Part model, mm, in its own coordinate system. A direction names the side the tool comes from. Round coordinates to 2 decimals unless told otherwise and drop trailing zeros. Loops run counter-clockwise (first coordinate to the right, second up) from the corner with the lowest first, then second, coordinate; pieces in that order, holes last.
from build123d import *

# Parameters (mm, degrees)
SKETCH_1_W           = 30
SKETCH_1_H           = 14.828427124
EXTRUDE_2_DEPTH      = 10
CUT_EXTRUDE_9_DEPTH  = 15
CUT_EXTRUDE_10_DEPTH = 30
CUT_EXTRUDE_11_DEPTH = 31
CUT_EXTRUDE_12_DEPTH = 40
SKETCH_1_15_R        = 6
CUT_EXTRUDE_13_DEPTH = 17
CUT_EXTRUDE_17_DEPTH = 97
CUT_EXTRUDE_18_DEPTH = 285
CUT_EXTRUDE_20_DEPTH = 202
CUT_EXTRUDE_21_DEPTH = 202
CUT_EXTRUDE_22_DEPTH = 95


with BuildPart() as part:
    # Sketch 1 → Extrude 2 (new body)
    with BuildSketch(Plane.XY):
        with Locations((7.585786438, 0)):
            Rectangle(SKETCH_1_W, SKETCH_1_H)
    extrude(amount=EXTRUDE_2_DEPTH)

    # Sketch 1_11 → Cut-Extrude 9 (cut)
    with BuildSketch(Plane.XY):
        with BuildLine():
            Line((0, -2), (0, 0))
            Line((0, 0), (-6, 0))
            ThreePointArc((-6, 0), (-4.242640687, -4.242640687), (0, -6))
            ThreePointArc((0, -6), (3.464101615, -4.898979486), (5.656854249, -2))
            Line((5.656854249, -2), (0, -2))
        make_face()
    extrude(amount=CUT_EXTRUDE_9_DEPTH, mode=Mode.SUBTRACT)

    # Sketch 1_12 → Cut-Extrude 10 (cut)
    with BuildSketch(Plane.XY):
        with BuildLine():
            Line((-6, 0), (0, 0))
            Line((0, 0), (0, 2))
            Line((0, 2), (0, 6))
            ThreePointArc((0, 6), (-4.242640687, 4.242640687), (-6, 0))
        make_face()
    extrude(amount=CUT_EXTRUDE_10_DEPTH, mode=Mode.SUBTRACT)

    # Sketch 1_13 → Cut-Extrude 11 (cut)
    with BuildSketch(Plane.XY):
        with BuildLine():
            Line((0, 2), (0, 0))
            Line((0, 0), (6, 0))
            ThreePointArc((6, 0), (5.913591358, 1.014611872), (5.656854249, 2))
            Line((5.656854249, 2), (0, 2))
        make_face()
    extrude(amount=CUT_EXTRUDE_11_DEPTH, mode=Mode.SUBTRACT)

    # Sketch 1_14 → Cut-Extrude 12 (cut)
    with BuildSketch(Plane.XY):
        with BuildLine():
            Line((6, 0), (0, 0))
            Line((0, 0), (0, -2))
            Line((0, -2), (5.656854249, -2))
            ThreePointArc((5.656854249, -2), (5.913591358, -1.014611872), (6, 0))
        make_face()
    extrude(amount=CUT_EXTRUDE_12_DEPTH, mode=Mode.SUBTRACT)

    # Sketch 1_15 → Cut-Extrude 13 (cut)
    with BuildSketch(Plane.XY):
        with Locations(Location((0, 0, 0), (0, 0, 180))):
            Circle(SKETCH_1_15_R)
    extrude(amount=CUT_EXTRUDE_13_DEPTH, mode=Mode.SUBTRACT)

    # Sketch 1_19 → Cut-Extrude 17 (cut)
    with BuildSketch(Plane.XY):
        with BuildLine():
            ThreePointArc((5.656854249, 2), (5.913591358, 1.014611872), (6, 0))
            Line((6, 0), (6, 2))
            Line((6, 2), (5.656854249, 2))
        make_face()
        Polygon((6, 2), (6, 0), (7, 0), (7, 1), (7, 2), align=None)
        Polygon((7, 0), (6, 0), (6, -2), (7, -2), (7, -1), align=None)
        with BuildLine():
            Line((6, -2), (6, 0))
            ThreePointArc((6, 0), (5.913591358, -1.014611872), (5.656854249, -2))
            Line((5.656854249, -2), (6, -2))
        make_face()
    extrude(amount=CUT_EXTRUDE_17_DEPTH, mode=Mode.SUBTRACT)

    # Sketch 1_20 → Cut-Extrude 18 (cut)
    with BuildSketch(Plane.XY):
        with BuildLine():
            ThreePointArc((7.414213562, 7.414213562), (9.005239827, 5.370919954), (10.046946078, 3))
            Line((10.046946078, 3), (18, 3))
            Line((18, 3), (18, 2))
            Line((18, 2), (18, 1))
            Line((18, 1), (18, -1))
            Line((18, -1), (18, -2))
            Line((18, -2), (18, -3))
            Line((18, -3), (10.046946078, -3))
            ThreePointArc((10.046946078, -3), (9.005239827, -5.370919954), (7.414213562, -7.414213562))
            Line((7.414213562, -7.414213562), (22.585786438, -7.414213562))
            Line((22.585786438, -7.414213562), (22.585786438, 7.414213562))
            Line((22.585786438, 7.414213562), (7.414213562, 7.414213562))
        make_face()
    extrude(amount=CUT_EXTRUDE_18_DEPTH, mode=Mode.SUBTRACT)

    # Sketch 1_22 → Cut-Extrude 20 (cut)
    with BuildSketch(Plane.XY):
        with BuildLine():
            ThreePointArc((10.485281374, 0), (10.473325852, -0.500570761), (10.437486551, -1))
            Line((10.437486551, -1), (18, -1))
            Line((18, -1), (18, 1))
            Line((18, 1), (10.437486551, 1))
            ThreePointArc((10.437486551, 1), (10.473325852, 0.500570761), (10.485281374, 0))
        make_face()
    extrude(amount=CUT_EXTRUDE_20_DEPTH, mode=Mode.SUBTRACT)

    # Sketch 2 → Cut-Extrude 21 (cut)
    with BuildSketch(Plane.XZ.offset(3)):
        with BuildLine():
            ThreePointArc((14.807762643, 5.986148983), (14.023473039, 6.26), (13.239183435, 5.986148983))
            Line((13.239183435, 5.986148983), (14.023473039, 5))
            Line((14.023473039, 5), (14.807762643, 5.986148983))
        make_face()
        with BuildLine():
            Line((14.023473039, 5), (13.239183435, 5.986148983))
            ThreePointArc((13.239183435, 5.986148983), (12.763473039, 5), (13.239183435, 4.013851017))
            Line((13.239183435, 4.013851017), (14.023473039, 5))
        make_face()
        with BuildLine():
            Line((14.807762643, 5.986148983), (14.023473039, 5))
            Line((14.023473039, 5), (14.807762643, 4.013851017))
            ThreePointArc((14.807762643, 4.013851017), (15.158330938, 4.45255361), (15.283473039, 5))
            ThreePointArc((15.283473039, 5), (15.158330938, 5.54744639), (14.807762643, 5.986148983))
        make_face()
        with BuildLine():
            Line((14.807762643, 4.013851017), (14.023473039, 5))
            Line((14.023473039, 5), (13.239183435, 4.013851017))
            ThreePointArc((13.239183435, 4.013851017), (14.023473039, 3.74), (14.807762643, 4.013851017))
        make_face()
    extrude(amount=-CUT_EXTRUDE_21_DEPTH, mode=Mode.SUBTRACT)

    # Sketch 1_23 → Cut-Extrude 22 (cut)
    with BuildSketch(Plane.XY):
        with BuildLine():
            Line((7, 1), (7, 0))
            Line((7, 0), (7, -1))
            Line((7, -1), (10.437486551, -1))
            ThreePointArc((10.437486551, -1), (10.473325852, -0.500570761), (10.485281374, 0))
            ThreePointArc((10.485281374, 0), (10.473325852, 0.500570761), (10.437486551, 1))
            Line((10.437486551, 1), (7, 1))
        make_face()
        with BuildLine():
            ThreePointArc((10.485281374, 0), (10.473325852, -0.500570761), (10.437486551, -1))
            Line((10.437486551, -1), (18, -1))
            Line((18, -1), (18, 1))
            Line((18, 1), (10.437486551, 1))
            ThreePointArc((10.437486551, 1), (10.473325852, 0.500570761), (10.485281374, 0))
        make_face()
    extrude(amount=CUT_EXTRUDE_22_DEPTH, mode=Mode.SUBTRACT)


solid = part.part
1) Slice it at A-A, the plane y = -2.75. Give the cut face in (x, z).
Values:
outline: (-7.41, 0) - (-5.33, 0) - (-5.33, 10) - (-7.41, 10) - close; (5.33, 0) - (18, 0) - (18, 10) - (5.33, 10) - close; hole circle Ø2.52 at (14.02, 5)
2) Tool access for faces 1 (the face through (8, 2, 0)), 2 (the face through (7, 1.5, 4.9)), 3 (the face through (14.9, 3, 3.8)), 4 (the face through (12.6, 1, 4.9)): list every direction of +Z, -Z, +X, -X, +Y, -Y with a clear straight run to the whole face (end or side of a thin tool).
Values:
face 1: -Z, +X, -X, +Y, -Y
face 2: +Z, -Z
face 3: +Z, -Z, +X, +Y
face 4: +Z, -Z, +X
3) Slice it at C-C, the plane y = -4.5. Give the cut face in (x, z), then the cut area to 3 significant figures.
Values:
outline: (-7.41, 0) - (-3.97, 0) - (-3.97, 10) - (-7.41, 10) - close; (3.97, 0) - (9.47, 0) - (9.47, 10) - (3.97, 10) - close
area: 89.5 mm2
4) Wall check: line 1 along Y through (x, z) = (6.75, 9.75); line 2 along Y through (x, z) = (14.5, 2.5); line 3 along X through (y, z) = (0, 4.5). Give the ranges that are in metal, low to high.
Values:
line 1: y = -7.41 to -2, 2 to 7.41
line 2: y = -3 to -1, 1 to 3
line 3: x = -7.41 to -6
5) Slice it at B-B, the plane x = -3. Give the cut face in (y, z).
Values:
outline: (-7.41, 0) - (-5.2, 0) - (-5.2, 10) - (-7.41, 10) - close; (5.2, 0) - (7.41, 0) - (7.41, 10) - (5.2, 10) - close
6) Drop flat-ended pins along their axis: pin 1 Ø3 at (x, z) = (10.5, 3) entering from +Y; pin 2 Ø4 at (x, z) = (14.5, 3) entering from +Y; pin 3 Ø3 at (x, y) = (-4.5, 5.5) entering from -Z; pin 4 Ø3 at (x, z) = (14, 5) entering from -Y. Give the stop position or say it passes through.
Values:
pin 1: stops at y = 5.38
pin 2: stops at y = 3
pin 3: stops at z = 0
pin 4: stops at y = -3
7) Slice it at D-D, the plane x = 14.5. Give the cut face in (y, z), then the cut area to 3 significant figures.
Values:
outline: (-3, 0) - (-1, 0) - (-1, 3.83) - (-3, 3.83) - close; (-3, 6.17) - (-1, 6.17) - (-1, 10) - (-3, 10) - close; (1, 0) - (3, 0) - (3, 3.83) - (1, 3.83) - close; (1, 6.17) - (3, 6.17) - (3, 10) - (1, 10) - close
area: 30.7 mm2
8) Mould opens along X. For faces 5 (the face through (13, -3, 4)), 6 (the face through (18, 2, 5)), 7 (the face through (7, -1.5, 4.9)) say: released by +X, released by -X, zero draft, split by the parting line, or undercut.
Values:
face 5: zero draft
face 6: released by +X
face 7: undercut
